Here's how the part is built. I have some questions about the finished solid (model axes, mm). A direction names the side the tool comes from. Coordinates: 2 decimals unless noted, no trailing zeros. Loops run counter-clockwise (first coordinate to the right, second up) from the corner with the lowest first, then second, coordinate; pieces in that order, holes last. Notation, with made-up numbers: (25, -23.75) -> (73, -23.75) arc R17 ccw to (73, -17.75) -> close; hole circle Ø11 at (-31.5, -7). An arc over 180 degrees is marked (long way). Answer as a JSON object with one key per item and string values. Group by question number.
1) I want a section at B-B (y = 19.05). Write out the boundary of the cut face in (x, z) (3 decimals), then the cut area to 3 significant figures.
2) If we mould it in two halves opening along X, with no side actions, what happens to faces 1 (the flat face through (0, -1, -5)), 2 (the flat face through (7, -3.175, -11)), 3 (the cylindrical face through (6.39, -1.61, -18.04)), 4 (the flat face through (15, -1, -5))? For each: +X half, -X half, draft (parallel to the pull), parting line (faces both ways), or undercut.
3) I want a section at A-A (x = 7.5). Write out the boundary of the cut face in (y, z) (3 decimals), then the cut area to 3 significant figures.
4) I need wall thicknesses on probe 1 along Y at (x, z) = (4, -20.5) (3 decimals); probe 2 along Z at (x, y) = (11, 0.25) (3 decimals); probe 3 along Z at (x, y) = (7.5, -2.1). Which ranges of each line are inside material? Lowest first, please. Write a range as [from, to].
5) I want a section at D-D (x = 5). Write out the boundary of the cut face in (y, z) (3 decimals), then the cut area to 3 significant figures.
6) I want a section at C-C (z = -19.05). Write out the boundary of the cut face in (x, y) (3 decimals).
7) Which directions (+Z, -Z, +X, -X, +Y, -Y) give clear straight access to the entire face, cutting with the end or side of a thin tool? Please do faces 5 (the flat face through (7, 23.05, 2)), 6 (the flat face through (7, 11, 0)).
8) I'm going to push flat-ended pins straight in: pin 1 (5 mm diameter, centred on x = 7.5, z = -19.05, fed in from +Y); pin 2 (5 mm diameter, centred on x = 8, y = 6.5, fed in from -Z); pin 3 (8 mm diameter, centred on y = 7, z = -6.5, fed in from +X). Where does each tip first touch, or does it pass through?
```python
from build123d import *

# Parameters (mm, degrees)
BOSS_EXTRUDE1_DEPTH = 15
FILLET2_R           = 3.175
SKETCH7_R           = 1.5
CUT_EXTRUDE4_DEPTH  = 3.175
SKETCH8_R           = 1.5
CUT_EXTRUDE5_DEPTH  = 3.175


with BuildPart() as part:
    # Sketch1 → Boss-Extrude1 (new body)
    with BuildSketch(Plane(origin=(0, 0, 0), x_dir=(0, 0, -1), z_dir=(1, 0, 0))):
        Polygon((-3.175, 23.05), (-3.175, -3.175), (23.05, -3.175), (23.05, 0), (0, 0), (0, 23.05), align=None)
    extrude(amount=BOSS_EXTRUDE1_DEPTH)

    # Fillet2
    fillet2_edges = [part.edges().sort_by_distance(p)[0] for p in [
        (7.5, -3.175, 3.175),
    ]]
    fillet(fillet2_edges, radius=FILLET2_R)

    # Sketch7 → Cut-Extrude4 (cut)
    with BuildSketch(Plane.XY.offset(3.175)):
        with Locations((7.5, 19.05)):
            Circle(SKETCH7_R)
    extrude(amount=-CUT_EXTRUDE4_DEPTH, mode=Mode.SUBTRACT)

    # Sketch8 → Cut-Extrude5 (cut)
    with BuildSketch(Plane.XZ.offset(3.175)):
        with Locations((7.5, -19.05)):
            Circle(SKETCH8_R)
    extrude(amount=-CUT_EXTRUDE5_DEPTH, mode=Mode.SUBTRACT)


solid = part.part
```
Determined:
{
 "1": {"outline": "(0, 0) -> (6, 0) -> (6, 3.175) -> (0, 3.175) -> close; (9, 0) -> (15, 0) -> (15, 3.175) -> (9, 3.175) -> close", "area": "38.1 mm^2"},
 "2": {"face 1": "-X half", "face 2": "draft", "face 3": "undercut", "face 4": "+X half"},
 "3": {"outline": "(-3.175, -23.05) -> (0, -23.05) -> (0, -20.55) -> (-3.175, -20.55) -> close; (-3.175, -17.55) -> (0, -17.55) -> (0, 0) -> (17.55, 0) -> (17.55, 3.175) -> (0, 3.175) arc R3.175 ccw to (-3.175, 0) -> close; (20.55, 0) -> (23.05, 0) -> (23.05, 3.175) -> (20.55, 3.175) -> close", "area": "135 mm^2"},
 "4": {"probe 1": "[-3.175, 0]", "probe 2": "[0, 3.175]", "probe 3": "[-23.05, -20.55], [-17.55, 2.38]"},
 "5": {"outline": "(-3.175, -23.05) -> (0, -23.05) -> (0, 0) -> (23.05, 0) -> (23.05, 3.175) -> (0, 3.175) arc R3.175 ccw to (-3.175, 0) -> close", "area": "154 mm^2"},
 "6": {"outline": "(0, -3.175) -> (6, -3.175) -> (6, 0) -> (0, 0) -> close; (9, -3.175) -> (15, -3.175) -> (15, 0) -> (9, 0) -> close"},
 "7": {"face 5": "+Z, -Z, +X, -X, +Y", "face 6": "-Z, +X, -X, +Y"},
 "8": {"pin 1": "y = 0", "pin 2": "z = 0", "pin 3": "through"}
}
